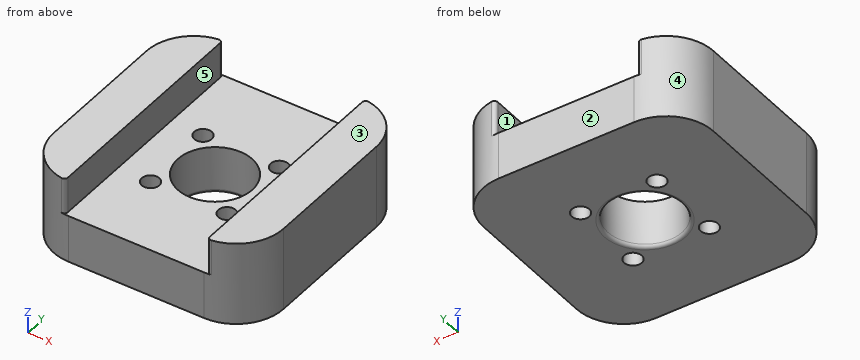
from build123d import *

# Parameters (mm, degrees)
F0_W     = 34
F0_H     = 34
F1_DEPTH = 12.3
F2_R     = 5.5
F3_DEPTH = 12.301
F4_R     = 1.3
F5_DEPTH = 12.301
F6_W     = 21
F6_H     = 5.3
F7_DEPTH = 34.001
F8_R     = 7
F9_R     = 0.5


with BuildPart() as f1:
    # F0 (on Top) → F1 (new body)
    with BuildSketch(Plane.XY):
        Rectangle(F0_W, F0_H)
    extrude(amount=F1_DEPTH)

    # F2 (on face) → F3 (cut, through all)
    with BuildSketch(Plane.XY.offset(12.3)):
        Circle(F2_R)
    extrude(amount=-F3_DEPTH, mode=Mode.SUBTRACT)

    # F4 (on face) → F5 (cut, through all)
    with BuildSketch(Plane(origin=(0, 0, 0), x_dir=(1, 0, 0), z_dir=(0, 0, -1))):
        with Locations((-5.65, 5.65)):
            Circle(F4_R)
        with Locations((-5.65, -5.65)):
            Circle(F4_R)
        with Locations((5.65, 5.65)):
            Circle(F4_R)
        with Locations((5.65, -5.65)):
            Circle(F4_R)
    extrude(amount=-F5_DEPTH, mode=Mode.SUBTRACT)

    # F6 (on face) → F7 (cut, through all)
    with BuildSketch(Plane.XZ.offset(17)):
        with Locations((0, 9.65)):
            Rectangle(F6_W, F6_H)
    extrude(amount=-F7_DEPTH, mode=Mode.SUBTRACT)

    # F8
    f8_edges = [f1.edges().sort_by_distance(p)[0] for p in [
        (-17, -17, 6.15),
        (17, -17, 6.15),
        (17, 17, 6.15),
        (-17, 17, 6.15),
    ]]
    fillet(f8_edges, radius=F8_R)

    # F9
    f9_edges = [f1.edges().sort_by_distance(p)[0] for p in [
        (-5.5, 0, 0),
        (-10.5, 16.98212, 9.65),
        (-10.5, -16.98212, 9.65),
        (10.5, -16.98212, 9.65),
        (10.5, 16.98212, 9.65),
    ]]
    fillet(f9_edges, radius=F9_R)


solid = f1.part
Geometry: final body of the model. Coordinates: model frame, mm. Face numbers are marked on the shaded views. A direction names the side the tool comes from. Round coordinates to 2 decimals unless told otherwise and drop trailing zeros. Loops run counter-clockwise (first coordinate to the right, second up) from the corner with the lowest first, then second, coordinate; pieces in that order, holes last. Notation, with made-up numbers: M -19.75,-17.75 L 9.25,-17.75 A25 ccw 9.25,0.25 Z; hole C 1,83 d7. An arc over 180 degrees is marked long. One line per question, with ' | ' between items.
(1) Cut plane B-B on z = 4.25. Return the cut outline in (x, y).
Check result:
outline: M -17,-10 A7 ccw -10,-17 L 10,-17 A7 ccw 17,-10 L 17,10 A7 ccw 10,17 L -10,17 A7 ccw -17,10 Z; hole C -5.65,-5.65 d2.6; hole C -5.65,5.65 d2.6; hole C 0,0 d11; hole C 5.65,-5.65 d2.6; hole C 5.65,5.65 d2.6
(2) Cut plane D-D on x = 13. Return the cut outline in (y, z).
Check result:
outline: M -16.32,0 L 16.32,0 L 16.32,12.3 L -16.32,12.3 Z
(3) Access query for the marked faces 1 and 2. Directions: +Z, -Z, +X, -X, +Y, -Y. A direction counts if a zero-diameter tool reaches every point of the face in a straight line with its end or side. Return the directions, or none.
Check result:
face 1: +Z, +Y, -Y | face 2: +Z, -Z, +X, -X, +Y
(4) Cut plane C-C on y = 8.5. Return the cut outline in (x, z), plus the area to 3 significant figures.
Check result:
outline: M -17,0 L 17,0 L 17,12.3 L 10.5,12.3 L 10.5,7 L -10.5,7 L -10.5,12.3 L -17,12.3 Z | area: 307 mm2
(5) Pull-direction query (X, two-part tool) for the marked faces 3, 4 and 5; classes: +X half, -X half, draft (parallel to the pull), parting line (faces both ways), or undercut.
Check result:
face 3: draft | face 4: -X half | face 5: undercut
(6) Cut plane A-A on y = 0. Return the cut outline in (x, z).
Check result:
outline: M -17,0 L -6,0 A0.5 ccw -5.5,0.5 L -5.5,7 L -10.5,7 L -10.5,12.3 L -17,12.3 Z; M 5.5,0.5 A0.5 ccw 6,0 L 17,0 L 17,12.3 L 10.5,12.3 L 10.5,7 L 5.5,7 Z
(7) Material intervals for line 1 along Y through (x, z) = (5.65, 4.25); line 2 along Y through (x, z) = (0, 3.25), sorted ascending. Write a range as from..to.
Check result:
line 1: y = -17..-6.95, -4.35..4.35, 6.95..17 | line 2: y = -17..-5.5, 5.5..17
(8) Contact query for flat-ended pins moving along their axis: P1, Ø4, axis at x = 5.65, y = 5.65, coming from the +Z side; P2, Ø4, axis at x = 13, z = 1.5, coming from the +Y side. Output: stop coordinate, or through.
Check result:
P1: stops at z = 7 | P2: stops at y = 16.93
